Solid Edge part; units mm, degrees
sketch "Sketch1" plane through (0, 0, 0) normal (0, 0, 1) x (1, 0, 0)
  circle A0 centre (0, 0) radius 14
extrude "Protrusion1" add sketch "Sketch1" along normal mid plane 10
hole "Bohrung_1" at (0, 0, 5) direction (0, 0, -1) diameter 12 end up to next
hole "Bohrung_2" at (0, 10.5, 5) direction (0, 0, -1) diameter 3 end up to next
pattern_circular "Pattern1" count 3 over 360 about axis through (0, 0, 5) along (0, 0, 1) of "Bohrung_2"
properties material "Wheel2"
Design review of the part built by this model. Coordinates are the model's own, in mm. Give positions to 0.01 mm unless a question says otherwise; leave off trailing zeros. Loops run counter-clockwise (first coordinate to the right, second up) from the corner with the lowest first, then second, coordinate; pieces in that order, holes last. Notation, with made-up numbers: (87, 6) - (138, 6) arc R31 cw to (138, 32) - close; hole circle Ø1 at (49.5, -35). An arc over 180 degrees is marked (long way). Use CSV: the item, a comma, the result in double quotes. Start each with the question number.
1. Wall thickness on L1, parallel to Y at x = 0, z = -1.75; L2, parallel to X at y = -5.25, z = 2; L3, parallel to X at y = -4.75, z = -2.25: over which ranges is each line inside the solid? List them lowest first.
2. Add section B-B (x = 0). State the section outline as (y, z) points, plus the area to 3 significant figures.
3. Add section D-D (x = -3). State the section outline as (y, z) points.
4. Draft analysis for pull direction Y (two halves, no side actions). For faces 1 (the flat face through (6, -3, -5)), 2 (the cylindrical face through (0, 6, 0)), 3 (the cylindrical face through (8.18, -4.06, 0.07)), 4 (the cylindrical face through (12.932, -5.362, 0.07)), state which applies: released by +Y, released by -Y, zero draft, split by the parting line, or undercut.
5. Insertion check: P1, Ø1, axis at y = 6.5, z = -2, coming from the -X side; P2, Ø1.5, axis at x = -2, z = -3.5, coming from the -Y side; P3, Ø3, axis at x = -2.5, z = 2, coming from the -Y side; P4, Ø2.5, axis at x = 0, y = 10.5, coming from the +Z side. Each pin has a flat end and moves straight along its axis. Give the tip position at first contact, or say it passes through.
6. Add section C-C (y = -5.25). State the section outline as (x, z) points, plus the area to 3 significant figures.
7. Add section A-A (y = 0). State the section outline as (x, z) points, plus the area to 3 significant figures.
Results found:
1,L1,"y = -14 to -6, 6 to 9, 12 to 14"
1,L2,"x = -12.98 to -10.59, -7.59 to -2.9, 2.9 to 7.59, 10.59 to 12.98"
1,L3,"x = -13.17 to -10.51, -7.68 to -3.67, 3.67 to 7.68, 10.51 to 13.17"
2,outline,"(-14, -5) - (-6, -5) - (-6, 5) - (-14, 5) - close; (6, -5) - (9, -5) - (9, 5) - (6, 5) - close; (12, -5) - (14, -5) - (14, 5) - (12, 5) - close"
2,area,"130 mm²"
3,outline,"(-13.67, -5) - (-5.2, -5) - (-5.2, 5) - (-13.67, 5) - close; (5.2, -5) - (13.67, -5) - (13.67, 5) - (5.2, 5) - close"
4,face 1,"zero draft"
4,face 2,"undercut"
4,face 3,"undercut"
4,face 4,"split by the parting line"
5,P1,"stops at x = -12.65"
5,P2,"stops at y = -13.94"
5,P3,"stops at y = -13.96"
5,P4,"passes through"
6,outline,"(-12.98, -5) - (-10.59, -5) - (-10.59, 5) - (-12.98, 5) - close; (-7.59, -5) - (-2.9, -5) - (-2.9, 5) - (-7.59, 5) - close; (2.9, -5) - (7.59, -5) - (7.59, 5) - (2.9, 5) - close; (10.59, -5) - (12.98, -5) - (12.98, 5) - (10.59, 5) - close"
6,area,"141 mm²"
7,outline,"(-14, -5) - (-6, -5) - (-6, 5) - (-14, 5) - close; (6, -5) - (14, -5) - (14, 5) - (6, 5) - close"
7,area,"160 mm²"
